Verification items for the finished model (mm, model axes). A direction names the side the tool comes from. Coordinates: 2 decimals unless noted, no trailing zeros. Loops run counter-clockwise (first coordinate to the right, second up) from the corner with the lowest first, then second, coordinate; pieces in that order, holes last. Notation, with made-up numbers: (-23.5, 68) - (8.5, 68) arc R19 cw to (8.5, 94) - close; hole circle Ø6 at (20.25, 6.25). An arc over 180 degrees is marked (long way). One line per item, written item: value. Start each with the question number.
(1) Gauge pin test, flat ends, axial feed: P1, Ø8.5, axis at x = 3.5, y = 18.5, coming from the -Z side; P2, Ø6.5, axis at x = 0, y = 20, coming from the -Z side (3 decimals). Record the tip position at first contact, or that the pin passes through.
(2) Draft check along X on faces 4 (the face through (0, 14, -6.35)), 5 (the face through (-39.688, 14, -6)), 6 (the face through (39.688, 14, -6)), 7 (the face through (-1, 14, 0)). Enter one of: +X half, -X half, draft (parallel to the pull), parting line (faces both ways), or undercut.
(3) Set-up check for faces 1 (the face through (3, 9, -3.175)), 2 (the face through (-15.888, 14, -9)), 3 (the face through (30.1, 15.27, -6.26)): record each of +Z, -Z, +X, -X, +Y, -Y from which the full face is reachable in a straight line by a thin tool's end or side.
(4) Thickness scan on probe 1 along Y at (x, z) = (0, -1.75) (3 decimals); probe 2 along X at (y, z) = (2.5, -10.5); probe 3 along X at (y, z) = (21.25, -4.5). Record the ranges inside material, lowest first. Write a range as [from, to].
(5) Section check A-A (x = 0). Record the boundary of the cut face in (y, z) (3 decimals), plus the area to 3 significant figures.
(6) Section check B-B (z = -8). Record the boundary of the cut face in (x, y) (1 decimal).
(7) Section check D-D (x = -26.5). Record the boundary of the cut face in (y, z) (3 decimals), plus the area to 3 significant figures.
```python
from build123d import *

# Parameters (mm, degrees)
BOSS_EXTRUDE1_DEPTH      = 28.575
F_5_16_18_TAPPED_HOLE1_D = 6.5278
HOLE4_D                  = 6.35
HOLE4_DEPTH              = 6.35
HOLE4_CBORE_D            = 12.7
HOLE4_CBORE_DEPTH        = 3.175
HOLE4_TIP                = 1.907732465


with BuildPart() as part:
    # Sketch1 → Boss-Extrude1 (new body)
    with BuildSketch(Plane(origin=(0, 0, 0), x_dir=(1, 0, 0), z_dir=(0, 1, 0))):
        Polygon((-39.6875, 0), (39.6875, 0), (39.6875, 12.7), (15.8877, 12.7), (15.8877, 6.35), (-15.8877, 6.35), (-15.8877, 12.7), (-39.6875, 12.7), align=None)
    extrude(amount=BOSS_EXTRUDE1_DEPTH)

    # 5/16-18 Tapped Hole1 (through all)
    with Locations(Plane(origin=(0, 0, -12.7), x_dir=(-1, 0, 0), z_dir=(0, 0, -1))):
        with Locations((26.9875, 14.2875), (-26.9875, 14.2875)):
            Hole(F_5_16_18_TAPPED_HOLE1_D / 2)

    # Hole4
    with Locations(Plane(origin=(0, 0, -6.35), x_dir=(-1, 0, 0), z_dir=(0, 0, -1))):
        with Locations((0, 21.1963), (0, 7.3787)):
            CounterBoreHole(HOLE4_D / 2, HOLE4_CBORE_D / 2, HOLE4_CBORE_DEPTH, depth=HOLE4_DEPTH)
            with Locations((0, 0, -(HOLE4_DEPTH + HOLE4_TIP / 2))):  # 118° drill point
                Cone(0, HOLE4_D / 2, HOLE4_TIP, mode=Mode.SUBTRACT)


solid = part.part
```
Responses:
1. P1: stops at z = -6.35
1. P2: stops at z = -3.175
2. face 4: undercut
2. face 5: -X half
2. face 6: +X half
2. face 7: draft
3. face 1: -Z
3. face 2: -Z, +Y, -Y
3. face 3: +Z, -Z
4. probe 1: y = [0, 4.204], [10.554, 18.021], [24.371, 28.575]
4. probe 2: x = [-39.69, -15.89], [15.89, 39.69]
4. probe 3: x = [-39.69, -6.35], [6.35, 39.69]
5. outline: (0, -6.35) - (1.029, -6.35) - (1.029, -3.175) - (4.204, -3.175) - (4.204, 0) - (0, 0) - close; (10.554, -3.175) - (13.729, -3.175) - (13.729, -6.35) - (14.846, -6.35) - (14.846, -3.175) - (18.021, -3.175) - (18.021, 0) - (10.554, 0) - close; (24.371, -3.175) - (27.546, -3.175) - (27.546, -6.35) - (28.575, -6.35) - (28.575, 0) - (24.371, 0) - close
5. area: 60.5 mm²
6. outline: (-39.7, 0) - (-15.9, 0) - (-15.9, 28.6) - (-39.7, 28.6) - close; (15.9, 0) - (39.7, 0) - (39.7, 28.6) - (15.9, 28.6) - close; hole circle Ø6.5 at (-27, 14.3); hole circle Ø6.5 at (27, 14.3)
7. outline: (0, -12.7) - (11.06, -12.7) - (11.06, 0) - (0, 0) - close; (17.515, -12.7) - (28.575, -12.7) - (28.575, 0) - (17.515, 0) - close
7. area: 281 mm²
